Source: three-view drawing plus pictorial views. Frame: mm from the lowest corner of the part. A direction names the side the tool comes from. Round coordinates to 2 decimals unless told otherwise and drop trailing zeros. Loops run counter-clockwise (first coordinate to the right, second up) from the corner with the lowest first, then second, coordinate; pieces in that order, holes last. Notation, with made-up numbers: (61, 64.25) -> (109, 64.25) arc R24 ccw to (109, 95.25) -> close; hole circle Ø7 at (16, 52). An arc over 180 degrees is marked (long way). Put each result on its own line as item: value. Start each with the question number.
1. Set-up query: the marked faces 1 and 2. Return all of +Z, -Z, +X, -X, +Y, -Y with unobstructed straight access to the full face (end or side cutting, diameter ignored); none if empty.
2. Material intervals for L1, parallel to X at y = 11.5, z = 8.5; L2, parallel to X at y = 5.25, z = 4.5 (1 decimal); L3, parallel to Z at x = 32.5, y = 7.5, sorted ascending.
3. Cut plane A-A (x = 16). Return the cut outline in (y, z) (1 decimal).
4. Contact query for flat-ended pins moving along their axis: pin 1 (3 mm diameter, centred on x = 38, z = 8.5, fed in from +Y); pin 2 (4 mm diameter, centred on x = 41, y = 6.5, fed in from -Z); pin 3 (2 mm diameter, centred on x = 127, z = 10.5, fed in from +Y). Output: stop coordinate, or through.
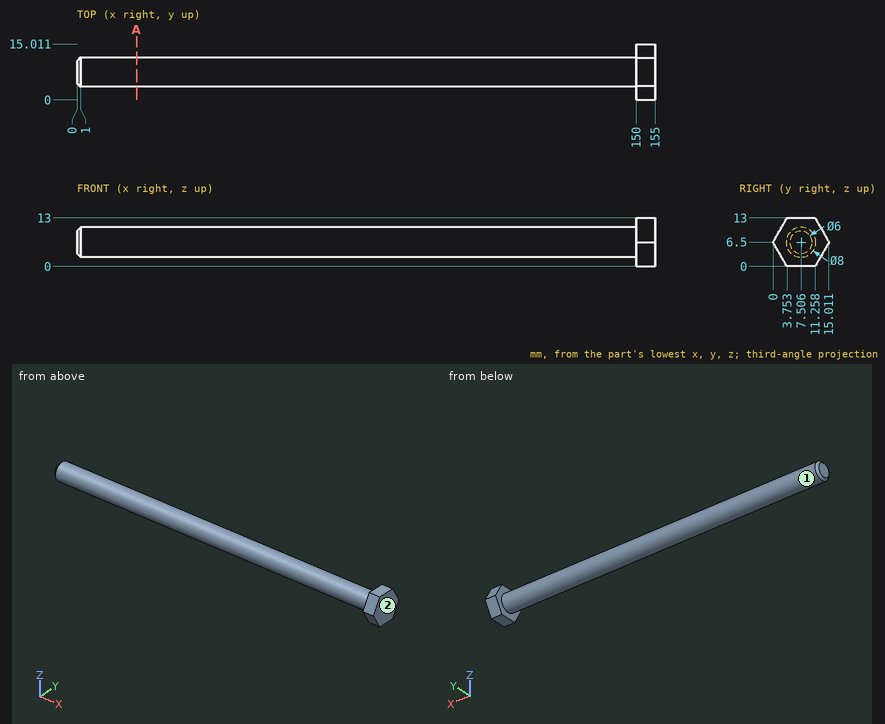
Solution:
1. face 1: -X
1. face 2: +Z, -Z, +X, +Y, -Y
2. L1: x = 150 to 155
2. L2: x = 0 to 155
2. L3: z = 2.5 to 10.5
3. outline: circle Ø8 at (7.5, 6.5)
4. pin 1: stops at y = 11.47
4. pin 2: stops at z = 2.5
4. pin 3: stops at y = 10.15
